The model under review builds one solid part; all positions refer to its coordinate system, in mm. Face numbers are marked on the shaded views. A direction names the side the tool comes from. Coordinates: 2 decimals unless noted, no trailing zeros. Write each loop counter-clockwise with the first axis right and the second up, starting at its lowest first coordinate (ties: lowest second). Pieces come first, ordered by that corner, then holes. Notation, with made-up numbers: (-19.75, 88.5) - (38.25, 88.5) arc R8 cw to (38.25, 103.5) - close; hole circle Ø5 at (31.5, -24.5). An arc over 180 degrees is marked (long way). Put each result on its own line as item: value.
from build123d import *

# Parameters (mm, degrees)
ESQUISSE1_W              = 30
ESQUISSE1_H              = 32
BOSS_EXTRU_2_DEPTH       = 77
ESQUISSE2_W              = 28
ESQUISSE2_H              = 68.8370016
ENL_V_MAT_EXTRU_4_DEPTH  = 30
ESQUISSE3_W              = 12
ESQUISSE3_H              = 9
ENL_V_MAT_EXTRU_5_DEPTH  = 87.884981441
ESQUISSE5_W              = 20
ESQUISSE5_H              = 4.856303455
BOSS_EXTRU_3_DEPTH       = 16
ESQUISSE6_W              = 12
ESQUISSE6_H              = 12
ENL_V_MAT_EXTRU_6_DEPTH  = 6
ESQUISSE7_W              = 30
ESQUISSE7_H              = 30
ENL_V_MAT_EXTRU_7_DEPTH  = 6
CONG_3_SIZE              = 5
CONG_3_SIZE_2            = 10
CONG_5_SIZE              = 5
CONG_5_SIZE_2            = 10
ESQUISSE10_W             = 4
ESQUISSE10_H             = 1
ENL_V_MAT_EXTRU_9_DEPTH  = 89.617154096
ESQUISSE16_R             = 3
ENL_V_MAT_EXTRU_11_DEPTH = 3
CONG_7_R                 = 1


with BuildPart() as part:
    # Esquisse1 → Boss.-Extru.2 (new body)
    with BuildSketch(Plane.XY):
        with Locations((15, 16)):
            Rectangle(ESQUISSE1_W, ESQUISSE1_H)
    extrude(amount=BOSS_EXTRU_2_DEPTH)

    # Esquisse2 → Enlèv. mat.-Extru.4 (cut)
    with BuildSketch(Plane(origin=(0, 32, 0), x_dir=(1, 0, 0), z_dir=(0, 1, 0))):
        with Locations((15, -36.4185008)):
            Rectangle(ESQUISSE2_W, ESQUISSE2_H)
    extrude(amount=-ENL_V_MAT_EXTRU_4_DEPTH, mode=Mode.SUBTRACT)

    # Esquisse3 → Enlèv. mat.-Extru.5 (cut, through all)
    with BuildSketch(Plane.XY.offset(2)):
        with Locations((15, 26.5)):
            Rectangle(ESQUISSE3_W, ESQUISSE3_H)
    extrude(amount=-ENL_V_MAT_EXTRU_5_DEPTH, mode=Mode.SUBTRACT)

    # Esquisse5 → Boss.-Extru.3 (add)
    with BuildSketch(Plane(origin=(0, 0, 0), x_dir=(-1, 0, 0), z_dir=(0, 0, -1))):
        with Locations((-16, 10.428151728)):
            Rectangle(ESQUISSE5_W, ESQUISSE5_H)
    extrude(amount=BOSS_EXTRU_3_DEPTH)

    # Esquisse6 → Enlèv. mat.-Extru.6 (cut)
    with BuildSketch(Plane(origin=(0, 12.856303455, 0), x_dir=(1, 0, 0), z_dir=(0, 1, 0))):
        with Locations((16, 6)):
            Rectangle(ESQUISSE6_W, ESQUISSE6_H)
    extrude(amount=-ENL_V_MAT_EXTRU_6_DEPTH, mode=Mode.SUBTRACT)

    # Esquisse7 → Enlèv. mat.-Extru.7 (cut)
    with BuildSketch(Plane.ZY):
        with Locations((55.8370016, 17)):
            Rectangle(ESQUISSE7_W, ESQUISSE7_H)
    extrude(amount=-ENL_V_MAT_EXTRU_7_DEPTH, mode=Mode.SUBTRACT)

    # Congé3
    # a fillet whose section is not a circle: 10, 5 mm, written as the material it takes off along each edge
    with BuildSketch(Plane(origin=(6, -17, -16), x_dir=(0, 0, 1), z_dir=(0, 1, 0))) as cong_3_piece_1:
        with BuildLine():
            Bezier((CONG_3_SIZE, 0), (0, 0), (0, CONG_3_SIZE_2), weights=[1, 0.707106781, 1])
            Line((0, CONG_3_SIZE_2), (0, 0))
            Line((0, 0), (CONG_3_SIZE, 0))
        make_face()
    extrude(amount=54.856303455, mode=Mode.SUBTRACT)

    # Congé5
    # a fillet whose section is not a circle: 10, 5 mm, written as the material it takes off along each edge
    with BuildSketch(Plane(origin=(26, 37.856303455, -16), x_dir=(0, 0, 1), z_dir=(0, -1, 0))) as cong_5_piece_1:
        with BuildLine():
            Bezier((CONG_5_SIZE, 0), (0, 0), (0, CONG_5_SIZE_2), weights=[1, 0.707106781, 1])
            Line((0, CONG_5_SIZE_2), (0, 0))
            Line((0, 0), (CONG_5_SIZE, 0))
        make_face()
    extrude(amount=54.856303455, mode=Mode.SUBTRACT)

    # Esquisse10 → Enlèv. mat.-Extru.9 (cut, through all)
    with BuildSketch(Plane(origin=(0, 0, 0), x_dir=(-1, 0, 0), z_dir=(0, 0, -1))):
        with Locations((-15, 0.5)):
            Rectangle(ESQUISSE10_W, ESQUISSE10_H)
    extrude(amount=-ENL_V_MAT_EXTRU_9_DEPTH, mode=Mode.SUBTRACT)

    # Esquisse16 → Enlèv. mat.-Extru.11 (cut)
    with BuildSketch(Plane.XY.offset(77)):
        with Locations((15, 10)):
            Circle(ESQUISSE16_R)
    extrude(amount=-ENL_V_MAT_EXTRU_11_DEPTH, mode=Mode.SUBTRACT)

    # Congé7
    cong_7_edges = [part.edges().sort_by_distance(p)[0] for p in [
        (21, 31, 1),
        (21, 22, 1),
        (9, 22, 1),
        (9, 31, 1),
    ]]
    fillet(cong_7_edges, radius=CONG_7_R)


solid = part.part
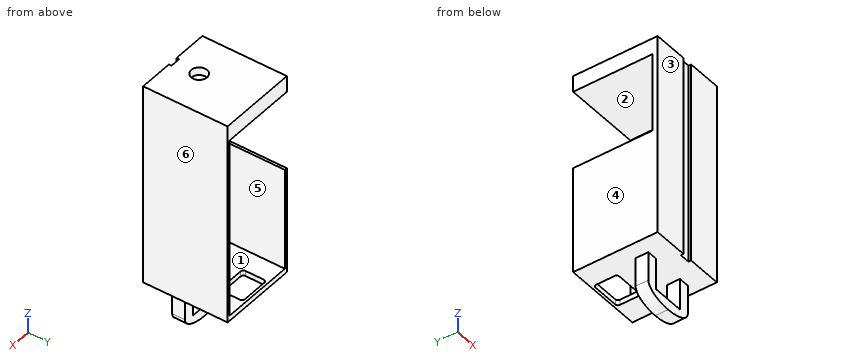
1. Consider section A-A on z = -4. State the section outline as (x, y) points, plus the area to 3 significant figures.
Determined:
outline: (6, 8) - (10, 8) - (10, 12.86) - (6, 12.86) - close; (22, 8) - (26, 8) - (26, 12.86) - (22, 12.86) - close
area: 38.9 mm^2
2. For pin 1 Ø6 at (x, y) = (15, 23) entering from -Z; pin 2 Ø10 at (x, z) = (22.5, 4.5) entering from -Y; pin 3 Ø2 at (x, z) = (14.5, 44.5) entering from -Y; pin 4 Ø2.5 at (y, z) = (11, -6.5) entering from +X, all flat-tipped, find the tip position at first contact; note any pin that passes through.
Determined:
pin 1: stops at z = 0
pin 2: stops at y = 0
pin 3: stops at y = 1
pin 4: stops at x = 26
3. To check wall thickness, follow probe 1 along X at (y, z) = (21, 14.5); probe 2 along Z at (x, y) = (28, 23); probe 3 along X at (y, z) = (12, -5.5). State the ranges of each line that lie inside material, in increasing order.
Determined:
probe 1: x = 0 to 1, 29 to 30
probe 2: z = 0 to 2, 70.84 to 77
probe 3: x = 6 to 10, 22 to 26
4. Consider section B-B on y = 25. State the section outline as (x, z) points, plus the area to 3 significant figures.
Determined:
outline: (0, 0) - (9, 0) - (9, 2) - (1, 2) - (1, 40.84) - (0, 40.84) - close; (0, 70.84) - (29, 70.84) - (29, 2) - (21, 2) - (21, 0) - (30, 0) - (30, 77) - (0, 77) - close
area: 329 mm^2
5. Consider section D-D on z = 60. State the section outline as (x, y) points.
Determined:
outline: (0, 0) - (13, 0) - (13, 1) - (17, 1) - (17, 0) - (30, 0) - (30, 32) - (29, 32) - (29, 2) - (0, 2) - close
6. Consider section C-C on x = 3.5. State the section outline as (y, z) points, plus the area to 3 significant figures.
Determined:
outline: (0, 0) - (32, 0) - (32, 2) - (2, 2) - (2, 70.84) - (32, 70.84) - (32, 77) - (0, 77) - close
area: 399 mm^2
7. The part is to be moulded in two halves that separate along X. For the marked faces 4, 5 and 6, say which applies: +X half, -X half, draft (parallel to the pull), parting line (faces both ways), or undercut.
Determined:
face 4: -X half
face 5: undercut
face 6: +X half
8. Machinability: for the marked faces 1, 2 and 3, which of the approach directions +Z, -Z, +X, -X, +Y, -Y give a long, thin tool a straight path to every point of the face, cutting with its end or side? Answer none if there is none.
Determined:
face 1: +Y
face 2: -X, +Y
face 3: +Z, -Z, +X, -X, -Y
